Geometry: final body of the model. Coordinates: model frame, mm. Give positions to 0.01 mm unless a question says otherwise; leave off trailing zeros. Order: outer loops, then holes, each group sorted by start corner. A loop starts at its lowest first (then second) coordinate and runs counter-clockwise, first axis right, second up. Notation, with made-up numbers: (73, -30) - (102, -30) arc R32 ccw to (102, 6) - close; hole circle Ø11 at (-6.75, 29.5). An arc over 180 degrees is marked (long way). Use one line per item in the form item = value.
from build123d import *

# Parameters (mm, degrees)
SKETCH6_R           = 2.1
BOSS_EXTRUDE1_DEPTH = 160


with BuildPart() as part:
    # Sketch6 → Boss-Extrude1 (new body)
    with BuildSketch(Plane.XY):
        with BuildLine():
            Line((-3.4, -2.339339828), (-3.4, 2.339339828))
            Line((-3.4, 2.339339828), (-6.560660172, 5.5))
            Line((-6.560660172, 5.5), (-8.2, 5.5))
            Line((-8.2, 5.5), (-8.2, 2.89))
            Line((-8.2, 2.89), (-8.31, 2.89))
            Line((-8.31, 2.89), (-9.768614357, 4.348614357))
            ThreePointArc((-9.768614357, 4.348614357), (-9.939864831, 4.604908803), (-10, 4.907228714))
            Line((-10, 4.907228714), (-10, 8.5))
            ThreePointArc((-10, 8.5), (-9.560660172, 9.560660172), (-8.5, 10))
            Line((-8.5, 10), (-4.907228714, 10))
            ThreePointArc((-4.907228714, 10), (-4.604908803, 9.939864831), (-4.348614357, 9.768614357))
            Line((-4.348614357, 9.768614357), (-2.89, 8.31))
            Line((-2.89, 8.31), (-2.89, 8.2))
            Line((-2.89, 8.2), (-5.5, 8.2))
            Line((-5.5, 8.2), (-5.5, 6.560660172))
            Line((-5.5, 6.560660172), (-2.339339828, 3.4))
            Line((-2.339339828, 3.4), (2.339339828, 3.4))
            Line((2.339339828, 3.4), (5.5, 6.560660172))
            Line((5.5, 6.560660172), (5.5, 8.2))
            Line((5.5, 8.2), (2.89, 8.2))
            Line((2.89, 8.2), (2.89, 8.31))
            Line((2.89, 8.31), (4.348614357, 9.768614357))
            ThreePointArc((4.348614357, 9.768614357), (4.604908803, 9.939864831), (4.907228714, 10))
            Line((4.907228714, 10), (8.5, 10))
            ThreePointArc((8.5, 10), (9.560660172, 9.560660172), (10, 8.5))
            Line((10, 8.5), (10, 4.907228714))
            ThreePointArc((10, 4.907228714), (9.939864831, 4.604908803), (9.768614357, 4.348614357))
            Line((9.768614357, 4.348614357), (8.31, 2.89))
            Line((8.31, 2.89), (8.2, 2.89))
            Line((8.2, 2.89), (8.2, 5.5))
            Line((8.2, 5.5), (6.560660172, 5.5))
            Line((6.560660172, 5.5), (3.4, 2.339339828))
            Line((3.4, 2.339339828), (3.4, -2.339339828))
            Line((3.4, -2.339339828), (6.560660172, -5.5))
            Line((6.560660172, -5.5), (8.2, -5.5))
            Line((8.2, -5.5), (8.2, -2.89))
            Line((8.2, -2.89), (8.31, -2.89))
            Line((8.31, -2.89), (9.768614357, -4.348614357))
            ThreePointArc((9.768614357, -4.348614357), (9.939864831, -4.604908803), (10, -4.907228714))
            Line((10, -4.907228714), (10, -8.5))
            ThreePointArc((10, -8.5), (9.560660172, -9.560660172), (8.5, -10))
            Line((8.5, -10), (4.907228714, -10))
            ThreePointArc((4.907228714, -10), (4.604908803, -9.939864831), (4.348614357, -9.768614357))
            Line((4.348614357, -9.768614357), (2.89, -8.31))
            Line((2.89, -8.31), (2.89, -8.2))
            Line((2.89, -8.2), (5.5, -8.2))
            Line((5.5, -8.2), (5.5, -6.560660172))
            Line((5.5, -6.560660172), (2.339339828, -3.4))
            Line((2.339339828, -3.4), (-2.339339828, -3.4))
            Line((-2.339339828, -3.4), (-5.5, -6.560660172))
            Line((-5.5, -6.560660172), (-5.5, -8.2))
            Line((-5.5, -8.2), (-2.89, -8.2))
            Line((-2.89, -8.2), (-2.89, -8.31))
            Line((-2.89, -8.31), (-4.348614357, -9.768614357))
            ThreePointArc((-4.348614357, -9.768614357), (-4.604908803, -9.939864831), (-4.907228714, -10))
            Line((-4.907228714, -10), (-8.5, -10))
            ThreePointArc((-8.5, -10), (-9.560660172, -9.560660172), (-10, -8.5))
            Line((-10, -8.5), (-10, -4.907228714))
            ThreePointArc((-10, -4.907228714), (-9.939864831, -4.604908803), (-9.768614357, -4.348614357))
            Line((-9.768614357, -4.348614357), (-8.31, -2.89))
            Line((-8.31, -2.89), (-8.2, -2.89))
            Line((-8.2, -2.89), (-8.2, -5.5))
            Line((-8.2, -5.5), (-6.560660172, -5.5))
            Line((-6.560660172, -5.5), (-3.4, -2.339339828))
        make_face()
        Circle(SKETCH6_R, mode=Mode.SUBTRACT)
        Polygon((-7.66, 6.57), (-6.57, 7.66), (-6.57, 8.2), (-8.2, 8.2), (-8.2, 6.57), align=None, mode=Mode.SUBTRACT)
        Polygon((8.2, 6.57), (7.66, 6.57), (6.57, 7.66), (6.57, 8.2), (8.2, 8.2), align=None, mode=Mode.SUBTRACT)
        Polygon((7.66, -6.57), (6.57, -7.66), (6.57, -8.2), (8.2, -8.2), (8.2, -6.57), align=None, mode=Mode.SUBTRACT)
        Polygon((-8.2, -6.57), (-7.66, -6.57), (-6.57, -7.66), (-6.57, -8.2), (-8.2, -8.2), align=None, mode=Mode.SUBTRACT)
    extrude(amount=-BOSS_EXTRUDE1_DEPTH)


solid = part.part
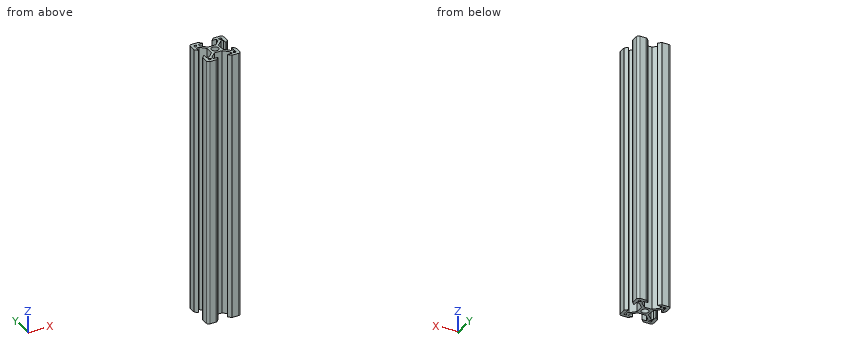
(1) Ray query, line 1 along X through (y, z) = (-8, -13.5); line 2 along Y through (x, z) = (0, -40.5); line 3 along Y through (x, z) = (-4.75, -63.5). Return the intervals inside material, ascending.
Computed values:
line_1 = -10 to -8.2, -6.57 to -5.5, 5.5 to 6.57, 8.2 to 10
line_2 = -3.4 to -2.1, 2.1 to 3.4
line_3 = -9.98 to -8.2, -5.81 to -3.69, 3.69 to 5.81, 8.2 to 9.98
(2) Cut plane A-A on x = 0. Output: boundary loops of the cut face in (y, z).
Computed values:
outline = (-3.4, -160) - (-2.1, -160) - (-2.1, 0) - (-3.4, 0) - close; (2.1, -160) - (3.4, -160) - (3.4, 0) - (2.1, 0) - close
(3) Cut plane C-C on z = -118. Give the number of separate pieces and of enclosed holes in the cut face, plus the area to 3 significant figures.
Computed values:
separate_pieces = 1
enclosed_holes = 5
area = 152 mm²
(4) Contact query for flat-ended pins moving along their axis: pin 1 Ø1.4 at (y, z) = (-0.5, -44.5) entering from +X; pin 2 Ø1 at (x, z) = (4, -102.5) entering from -Y; pin 3 Ø1.5 at (x, z) = (1, -131.5) entering from +Y. Output: stop coordinate, or through.
Computed values:
pin_1 = 3.4
pin_2 = -9.89
pin_3 = 3.4
